Check sheet for the modelled part. Datum: model origin and axes. Units: mm. Round coordinates to 2 decimals unless told otherwise and drop trailing zeros. Write each loop counter-clockwise with the first axis right and the second up, starting at its lowest first coordinate (ties: lowest second). Pieces come first, ordered by that corner, then holes.
Item 1: Section check A-A, the plane z = 6.25. Record the cut outline in (x, y) (1 decimal).
Item 2: Section check B-B, the plane y = 259.5. Record the cut outline in (x, z), plus the area to 3 significant figures.
Item 3: Material ranges on line 1 along Y through (x, z) = (46.5, 3.5); line 2 along Y through (x, z) = (49.5, 5.25); line 3 along Y through (x, z) = (68.5, 1.25), recorded low to high.
Item 4: Section check C-C, the plane x = 140.5. Record the cut outline in (y, z).
Item 5: Depth check by flat-ended pin: pin 1 (1 mm diameter, centred on y = 293, z = 3.5, fed in from +X); pin 2 (2.5 mm diameter, centred on x = 156.96, y = 108.31, fed in from -Z); pin 3 (1 mm diameter, centred on x = 159.5, z = 4.5, fed in from -Y); pin 4 (1.5 mm diameter, centred on x = 146, z = 5.5, fed in from +Y). Enter the tip coordinate at first touch or a pass-through.
Autodesk Inventor part; units mm, degrees
ref_plane "YZ Plane" through (0, 0, 0) normal (1, 0, 0) x (0, 1, 0)
ref_plane "XZ Plane" through (0, 0, 0) normal (0, 1, 0) x (-1, 0, 0)
ref_plane "XY Plane" through (0, 0, 0) normal (0, 0, 1) x (1, 0, 0)
sketch "Sketch1" plane through (0, 0, 0) normal (0, 0, 1) x (1, 0, 0)
  circle A0 centre (156.9617, 108.3117) radius 2.1844
  line L0 (171.7435, 196.3872) -> (150.4677, 101.0806)
  arc A1 (171.7435, 196.3872) -> (41.593, 297.4287) centre (78.8791, 211.1131) ccw
  arc A2 (152.3136, 109.3493) -> (161.5702, 107.1104) centre (156.9617, 108.3117) ccw
  line L1 (150.4677, 101.0806) -> (158.4911, 103.8014)
  line L2 (180.8293, 193.3835) -> (161.5702, 107.1104)
  circle A3 centre (40.3856, 300.9489) radius 2.1844
  arc A4 (180.8293, 193.3835) -> (38.7207, 304.2652) centre (83.4742, 215.1165) ccw
  arc A5 (56.9002, 306.3451) -> (27.9409, 294.5249) centre (78.8791, 211.1131) ccw construction
  arc A6 (56.4089, 308.4736) -> (39.5252, 302.9567) centre (78.8791, 211.1131) ccw
  arc A7 (57.3914, 304.2167) -> (41.2459, 298.941) centre (78.8791, 211.1131) ccw
  arc A8 (57.3914, 304.2167) -> (56.4089, 308.4736) centre (56.9002, 306.3451) ccw
  arc A9 (39.5252, 302.9567) -> (41.2459, 298.941) centre (40.3856, 300.9489) ccw
  line L3 (83.4742, 215.1165) -> (56.9002, 306.3451) construction
  arc A10 (41.5411, 297.4113) -> (41.593, 297.4287) centre (40.3856, 300.9489) ccw
  line L4 (40.3856, 300.9489) -> (84.3253, 219.1399) construction
  arc A11 (38.7207, 304.2652) -> (42.1414, 297.6798) centre (40.3856, 300.9489) ccw
  line L5 (171.7435, 196.3872) -> (180.8293, 193.3835) construction
  point P0 (0, 0)
  point P1 (165.3829, 124.1896)
  point P2 (27.4473, 296.7796)
  point P3 (41.1972, 299.4378)
  point P4 (41.8471, 297.538)
  point P5 (41.2459, 298.941)
  point P6 (39.5252, 302.9567)
  dimension "d0" = 9.525
  dimension "d1" = 0
  dimension "d7" = 12
extrude "Extrusion1" add sketch "Sketch1" along normal blind 7.62
fillet "Fillet1" radius 1 1 edges at (150.4677, 101.0806, 3.81)
properties part number "front rails" material "Acetal Resin, Black"
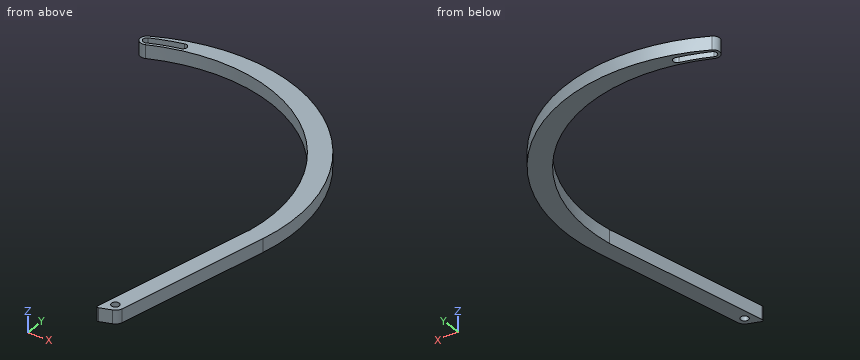
Values found:
1. outline: (38.7, 304.3) arc R3.7 ccw to (41.8, 297.5) arc R94 cw to (171.7, 196.4) - (150.9, 102.8) arc R1 ccw to (152.2, 101.7) - (158.5, 103.8) arc R4.8 ccw to (161.6, 107.1) - (180.8, 193.4) arc R99.8 ccw to start; hole (39.5, 303) arc R2.2 ccw to (41.2, 298.9) arc R95.5 cw to (57.4, 304.2) arc R2.2 ccw to (56.4, 308.5) arc R99.9 ccw to start; hole circle Ø4.4 at (157, 108.3)
2. outline: (159.5, 0) - (172.81, 0) - (172.81, 7.62) - (159.5, 7.62) - close
2. area: 101 mm2
3. line 1: y = 299.39 to 301.01, 305.64 to 307.76
3. line 2: y = 300.43 to 302.04, 306.62 to 308.9
3. line 3: y = 304.56 to 313.74
4. outline: (282.13, 0) - (296.96, 0) - (296.96, 7.62) - (282.13, 7.62) - close
5. pin 1: stops at x = 146.42
5. pin 2: passes through
5. pin 3: stops at y = 104.01
5. pin 4: stops at y = 293.44
